For this review, take the finished solid that the model builds, in its own axes (mm). A direction names the side the tool comes from. Give positions to 0.01 mm unless a question says otherwise; leave off trailing zeros. Order: outer loops, then holes, each group sorted by start corner. A loop starts at its lowest first (then second) coordinate and runs counter-clockwise, first axis right, second up.
from build123d import *

# Parameters (mm, degrees)
SKETCH1_R           = 1.25
BOSS_EXTRUDE1_DEPTH = 2.5
BOSS_EXTRUDE2_START = -2.5
BOSS_EXTRUDE2_DEPTH = 2.5
SKETCH3_R           = 1.5
CUT_EXTRUDE1_DEPTH  = 2.5


with BuildPart() as part:
    # Sketch1 → Boss-Extrude1 (new body)
    with BuildSketch(Plane(origin=(0, 0, 0), x_dir=(1, 0, 0), z_dir=(0, 1, 0))):
        with BuildLine():
            Line((-12, 101.75), (-12, 66.75))
            ThreePointArc((-12, 66.75), (-28.03590373, 28.03590373), (-66.75, 12))
            Line((-66.75, 12), (-101.75, 12))
            Line((-101.75, 12), (-101.75, -12))
            Line((-101.75, -12), (-66.75, -12))
            ThreePointArc((-66.75, -12), (-28.03590373, -28.03590373), (-12, -66.75))
            Line((-12, -66.75), (-12, -101.75))
            Line((-12, -101.75), (12, -101.75))
            Line((12, -101.75), (12, -66.75))
            ThreePointArc((12, -66.75), (28.03590373, -28.03590373), (66.75, -12))
            Line((66.75, -12), (101.75, -12))
            Line((101.75, -12), (101.75, 12))
            Line((101.75, 12), (66.75, 12))
            ThreePointArc((66.75, 12), (28.03590373, 28.03590373), (12, 66.75))
            Line((12, 66.75), (12, 101.75))
            Line((12, 101.75), (-12, 101.75))
        make_face()
        with Locations(Location((-7.75, 98.75, 0), (0, 0, 270))):
            Circle(SKETCH1_R, mode=Mode.SUBTRACT)
        with Locations(Location((7.75, 98.75, 0), (0, 0, 270))):
            Circle(SKETCH1_R, mode=Mode.SUBTRACT)
        with Locations(Location((7.75, -98.75, 0), (0, 0, 270))):
            Circle(SKETCH1_R, mode=Mode.SUBTRACT)
        with Locations(Location((-7.75, -98.75, 0), (0, 0, 270))):
            Circle(SKETCH1_R, mode=Mode.SUBTRACT)
        with Locations(Location((98.75, 7.75, 0), (0, 0, 270))):
            Circle(SKETCH1_R, mode=Mode.SUBTRACT)
        with Locations(Location((98.75, -7.75, 0), (0, 0, 270))):
            Circle(SKETCH1_R, mode=Mode.SUBTRACT)
        with Locations(Location((-98.75, -7.75, 0), (0, 0, 270))):
            Circle(SKETCH1_R, mode=Mode.SUBTRACT)
        with Locations(Location((-98.75, 7.75, 0), (0, 0, 270))):
            Circle(SKETCH1_R, mode=Mode.SUBTRACT)
        with BuildLine():
            ThreePointArc((-8.929765886, -37.605823446), (-20.964835918, -20.964835918), (-37.605823446, -8.929765886))
            ThreePointArc((-37.605823446, -8.929765886), (-43.104792317, 0), (-37.605823446, 8.929765886))
            ThreePointArc((-37.605823446, 8.929765886), (-20.964835918, 20.964835918), (-8.929765886, 37.605823446))
            ThreePointArc((-8.929765886, 37.605823446), (0, 43.104792317), (8.929765886, 37.605823446))
            ThreePointArc((8.929765886, 37.605823446), (20.964835918, 20.964835918), (37.605823446, 8.929765886))
            ThreePointArc((37.605823446, 8.929765886), (43.104792317, 0), (37.605823446, -8.929765886))
            ThreePointArc((37.605823446, -8.929765886), (20.964835918, -20.964835918), (8.929765886, -37.605823446))
            ThreePointArc((8.929765886, -37.605823446), (0, -43.104792317), (-8.929765886, -37.605823446))
        make_face(mode=Mode.SUBTRACT)
    extrude(amount=BOSS_EXTRUDE1_DEPTH)

    # Sketch2 → Boss-Extrude2 (add)
    with BuildSketch(Plane(origin=(0, 2.5, 0), x_dir=(1, 0, 0), z_dir=(0, 1, 0)).offset(BOSS_EXTRUDE2_START)):
        with BuildLine():
            ThreePointArc((-18.108940598, -24.011143671), (-17.840648159, -23.148674772), (-17.75, -22.25))
            ThreePointArc((-17.75, -22.25), (-19.767576438, -18.496658387), (-24.011143671, -18.108940598))
            ThreePointArc((-24.011143671, -18.108940598), (-20.964835918, -20.964835918), (-18.108940598, -24.011143671))
        make_face()
        with BuildLine():
            ThreePointArc((-24.011143671, 18.108940598), (-19.767576438, 18.496658387), (-17.75, 22.25))
            ThreePointArc((-17.75, 22.25), (-17.840648159, 23.148674772), (-18.108940598, 24.011143671))
            ThreePointArc((-18.108940598, 24.011143671), (-20.964835918, 20.964835918), (-24.011143671, 18.108940598))
        make_face()
        with BuildLine():
            ThreePointArc((24.011143671, 18.108940598), (20.964835918, 20.964835918), (18.108940598, 24.011143671))
            ThreePointArc((18.108940598, 24.011143671), (19.068019485, 19.068019485), (24.011143671, 18.108940598))
        make_face()
        with BuildLine():
            ThreePointArc((18.108940598, -24.011143671), (20.964835918, -20.964835918), (24.011143671, -18.108940598))
            ThreePointArc((24.011143671, -18.108940598), (19.068019485, -19.068019485), (18.108940598, -24.011143671))
        make_face()
    extrude(amount=BOSS_EXTRUDE2_DEPTH)

    # Sketch3 → Cut-Extrude1 (cut)
    with BuildSketch(Plane(origin=(0, 2.5, 0), x_dir=(1, 0, 0), z_dir=(0, 1, 0))):
        with Locations(Location((-22.25, 22.25, 0), (0, 0, 270))):
            Circle(SKETCH3_R)
        with Locations(Location((22.25, 22.25, 0), (0, 0, 270))):
            Circle(SKETCH3_R)
        with Locations(Location((22.25, -22.25, 0), (0, 0, 270))):
            Circle(SKETCH3_R)
        with Locations(Location((-22.25, -22.25, 0), (0, 0, 270))):
            Circle(SKETCH3_R)
    extrude(amount=-CUT_EXTRUDE1_DEPTH, mode=Mode.SUBTRACT)


solid = part.part
1) Draft analysis for pull direction X (two halves, no side actions). For faces 1 (the face through (13.023, 1.232, -30.612)), 2 (the face through (-27.613, 1.232, -28.464)), 3 (the face through (-16, 0, 30)), 4 (the face through (27.613, 1.232, 28.464)), state which applies: +X half, -X half, draft (parallel to the pull), parting line (faces both ways), or undercut.
Answer sheet:
face 1: undercut
face 2: -X half
face 3: draft
face 4: +X half
2) We need section C-C on z = -48.5. Give the boundary of the cut face in (x, y), then the cut area to 3 significant figures.
Answer sheet:
outline: (-15.13, 0) - (15.13, 0) - (15.13, 2.5) - (-15.13, 2.5) - close
area: 75.7 mm2
3) Clearance check with flat-ended pins moving along their axes: pin 1 (2 mm diameter, centred on x = 7.75, z = -98.75, fed in from -Y); pin 2 (1.2 mm diameter, centred on y = 2, z = 77, fed in from -X); pin 3 (0.8 mm diameter, centred on y = 1.5, z = -85, fed in from +X); pin 4 (1 mm diameter, centred on x = 61.5, y = 2, fed in from +Z). State where each tip first meets the part, or that it passes through.
Answer sheet:
pin 1: passes through
pin 2: stops at x = -12
pin 3: stops at x = 12
pin 4: stops at z = 12.3
4) To check wall thickness, follow line 1 (X direction, y = 1.45, z = 98.75); line 2 (X direction, y = 1.7, z = -22.25). State the ranges of each line that lie inside material, in increasing order.
Answer sheet:
line 1: x = -12 to -9, -6.5 to 6.5, 9 to 12
line 2: x = -34.85 to -23.75, -20.75 to -17.75, 17.75 to 20.75, 23.75 to 34.85
5) We need section A-A on y = 0.65. Count the separate pieces of the cut face and the enclosed holes in it, then the cut area to 3 significant figures.
Answer sheet:
separate pieces: 1
enclosed holes: 13
area: 7,820 mm2
6) Tool access review of faces 5 (the face through (-0.155, 1.232, -43.104)), 6 (the face through (28.464, 1.232, -27.613)): name each direction out of +Z, -Z, +X, -X, +Y, -Y from which nothing blocks a thin tool from reaching the whole face with its end or side.
Answer sheet:
face 5: +Y, -Y
face 6: -Z, +X, +Y, -Y
7) We need section B-B on x = -77. Give the boundary of the cut face in (y, z).
Answer sheet:
outline: (0, -12) - (2.5, -12) - (2.5, 12) - (0, 12) - close
